The drawing under review shows one solid part. Ordinate dimensions are in mm from its lowest x, y, z. A direction names the side the tool comes from. Give positions to 0.01 mm unless a question says otherwise; leave off trailing zeros. Order: outer loops, then holes, each group sorted by start corner. A loop starts at its lowest first (then second) coordinate and runs counter-clockwise, first axis right, second up. Notation, with made-up numbers: M -28.75,19.25 L -3.75,19.25 A24 cw -3.75,43.25 Z; hole C 3,76 d11. An arc over 180 degrees is marked long. Put each result on its own line as item: value. Start each with the question number.
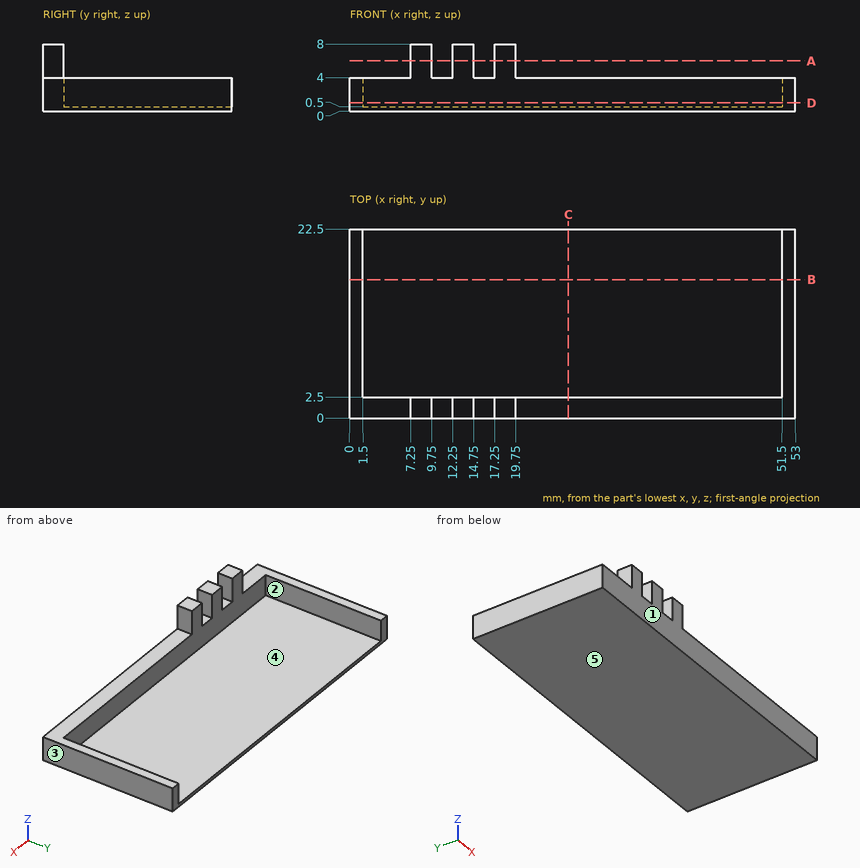
1. Consider section C-C on x = 26. Give the boundary of the cut face in (y, z).
2. Consider section D-D on z = 1. Give the boundary of the cut face in (x, y), then the cut area to 4 significant figures.
3. The part is to be moulded in two halves that separate along X. For the marked faces 1, 2 and 3, say which applies: +X half, -X half, draft (parallel to the pull), parting line (faces both ways), or undercut.
4. Consider section A-A on z = 6. Give the boundary of the cut face in (x, y), then the cut area to 4 significant figures.
5. Consider section B-B on y = 16.5. Give the boundary of the cut face in (x, z).
6. Machinability: for the marked faces 4 and 5, which of the approach directions +Z, -Z, +X, -X, +Y, -Y give a long, thin tool a straight path to every point of the face, cutting with its end or side? Answer none if there is none.
7. To check wall thickness, follow probe 1 along X at (y, z) = (15.5, 3.75); probe 2 along Z at (x, y) = (14.5, 18.5); probe 3 along Y at (x, z) = (5, 2.5). State the ranges of each line that lie inside material, in increasing order.
8. Insertion check: pin 1 (0.8 mm diameter, centred on x = 11, y = 1.5, fed in from +Z); pin 2 (0.8 mm diameter, centred on y = 1.5, z = 6, fed in from +X); pin 3 (10 mm diameter, centred on x = 8.5, y = 20, fed in from +Z). Each pin has a flat end and moves straight along its axis. Give the tip position at first contact, or say it passes through.
Returned:
1. outline: M 0,0 L 22.5,0 L 22.5,0.5 L 2.5,0.5 L 2.5,4 L 0,4 Z
2. outline: M 0,0 L 53,0 L 53,22.5 L 51.5,22.5 L 51.5,2.5 L 1.5,2.5 L 1.5,22.5 L 0,22.5 Z
2. area: 192.5 mm2
3. face 1: draft
3. face 2: undercut
3. face 3: +X half
4. outline: M 7.25,0 L 9.75,0 L 9.75,2.5 L 7.25,2.5 Z; M 12.25,0 L 14.75,0 L 14.75,2.5 L 12.25,2.5 Z; M 17.25,0 L 19.75,0 L 19.75,2.5 L 17.25,2.5 Z
4. area: 18.75 mm2
5. outline: M 0,0 L 53,0 L 53,4 L 51.5,4 L 51.5,0.5 L 1.5,0.5 L 1.5,4 L 0,4 Z
6. face 4: +Z, +Y
6. face 5: -Z, +X, -X, +Y, -Y
7. probe 1: x = 0 to 1.5, 51.5 to 53
7. probe 2: z = 0 to 0.5
7. probe 3: y = 0 to 2.5
8. pin 1: stops at z = 4
8. pin 2: stops at x = 19.75
8. pin 3: stops at z = 0.5
